```python
from build123d import *

# Parameters (mm, degrees)
SKETCH_1_W                = 54
SKETCH_1_H                = 220
EXTRUDE_1_DEPTH           = 30
SKETCH_2_W                = 42.2
SKETCH_2_H                = 48
CUT_EXTRUDE_1_DEPTH       = 25
SKETCH_3_W                = 42.2
SKETCH_3_H                = 46
CUT_EXTRUDE_2_DEPTH       = 25
CUT_EXTRUDE_3_DEPTH       = 6
CUT_EXTRUDE_13_DEPTH      = 6
SKETCH_18_W               = 32.2
SKETCH_18_H               = 32.2
CUT_EXTRUDE_9_DEPTH       = 6
SKETCH_9_R                = 15.6
SKETCH_9_R_2              = 1.6
CUT_EXTRUDE_4_DEPTH       = 25
SKETCH_16_W               = 42.7
SKETCH_16_H               = 42.7
CUT_EXTRUDE_7_DEPTH       = 2.5
SKETCH_13_R               = 20.35
SKETCH_13_R_2             = 2.1
CUT_EXTRUDE_6_DEPTH       = 28.5
EXTRUDE_3_DEPTH           = 30
SKETCH_17_R               = 1.5
CUT_EXTRUDE_8_DEPTH       = 8
SKETCH_21_R               = 3.5
CUT_EXTRUDE_11_DEPTH      = 1
CUT_EXTRUDE_11_DEPTH_BACK = 7.5
EXTRUDE_4_DEPTH           = 30
SKETCH_29_R               = 3
CUT_EXTRUDE_15_DEPTH      = 3
SKETCH_30_R               = 1.5
CUT_EXTRUDE_16_DEPTH      = 8


with BuildPart() as part:
    # 草图1 → 凸台-拉伸1 (new body)
    with BuildSketch(Plane.XY):
        Rectangle(SKETCH_1_W, SKETCH_1_H)
    extrude(amount=EXTRUDE_1_DEPTH)

    # 草图2 → 切除-拉伸1 (cut)
    with BuildSketch(Plane.XY.offset(30)):
        with Locations((0, 33)):
            Rectangle(SKETCH_2_W, SKETCH_2_H)
    extrude(amount=-CUT_EXTRUDE_1_DEPTH, mode=Mode.SUBTRACT)

    # 草图3 → 切除-拉伸2 (cut)
    with BuildSketch(Plane(origin=(0, 0, 30), x_dir=(-1, 0, 0), z_dir=(0, 0, -1))):
        with Locations((0, -33)):
            Rectangle(SKETCH_3_W, SKETCH_3_H)
    extrude(amount=CUT_EXTRUDE_2_DEPTH, mode=Mode.SUBTRACT)

    # 草图4 → 切除-拉伸3 (cut, through all)
    with BuildSketch(Plane.XY.offset(5)):
        with BuildLine():
            Line((11, 31), (11, 35))
            ThreePointArc((11, 35), (0, 46), (-11, 35))
            Line((-11, 35), (-11, 31))
            ThreePointArc((-11, 31), (0, 20), (11, 31))
        make_face()
        with BuildLine():
            Line((-14, 46.5), (-14, 50.5))
            ThreePointArc((-14, 50.5), (-15.5, 52), (-17, 50.5))
            Line((-17, 50.5), (-17, 46.5))
            ThreePointArc((-17, 46.5), (-15.5, 45), (-14, 46.5))
        make_face()
        with BuildLine():
            ThreePointArc((17, 50.5), (15.5, 52), (14, 50.5))
            Line((14, 50.5), (14, 46.5))
            ThreePointArc((14, 46.5), (15.5, 45), (17, 46.5))
            Line((17, 46.5), (17, 50.5))
        make_face()
        with BuildLine():
            Line((14, 19.5), (14, 15.5))
            ThreePointArc((14, 15.5), (15.5, 14), (17, 15.5))
            Line((17, 15.5), (17, 19.5))
            ThreePointArc((17, 19.5), (15.5, 21), (14, 19.5))
        make_face()
        with BuildLine():
            ThreePointArc((-17, 15.5), (-15.5, 14), (-14, 15.5))
            Line((-14, 15.5), (-14, 19.5))
            ThreePointArc((-14, 19.5), (-15.5, 21), (-17, 19.5))
            Line((-17, 19.5), (-17, 15.5))
        make_face()
    extrude(amount=-CUT_EXTRUDE_3_DEPTH, mode=Mode.SUBTRACT)

    # 草图26 → 切除-拉伸13 (cut, through all)
    with BuildSketch(Plane.XY.offset(5)):
        with BuildLine():
            Line((11, -31), (11, -35))
            ThreePointArc((11, -35), (0, -46), (-11, -35))
            Line((-11, -35), (-11, -31))
            ThreePointArc((-11, -31), (0, -20), (11, -31))
        make_face()
        with BuildLine():
            Line((-13.95, -15.5), (-13.95, -19.5))
            ThreePointArc((-13.95, -19.5), (-15.5, -21.05), (-17.05, -19.5))
            Line((-17.05, -19.5), (-17.05, -15.5))
            ThreePointArc((-17.05, -15.5), (-15.5, -13.95), (-13.95, -15.5))
        make_face()
        with BuildLine():
            Line((-13.95, -50.5), (-13.95, -46.5))
            ThreePointArc((-13.95, -46.5), (-15.5, -44.95), (-17.05, -46.5))
            Line((-17.05, -46.5), (-17.05, -50.5))
            ThreePointArc((-17.05, -50.5), (-15.5, -52.05), (-13.95, -50.5))
        make_face()
        with BuildLine():
            Line((13.95, -50.5), (13.95, -46.5))
            ThreePointArc((13.95, -46.5), (15.5, -44.95), (17.05, -46.5))
            Line((17.05, -46.5), (17.05, -50.5))
            ThreePointArc((17.05, -50.5), (15.5, -52.05), (13.95, -50.5))
        make_face()
        with BuildLine():
            Line((13.95, -15.5), (13.95, -19.5))
            ThreePointArc((13.95, -19.5), (15.5, -21.05), (17.05, -19.5))
            Line((17.05, -19.5), (17.05, -15.5))
            ThreePointArc((17.05, -15.5), (15.5, -13.95), (13.95, -15.5))
        make_face()
    extrude(amount=-CUT_EXTRUDE_13_DEPTH, mode=Mode.SUBTRACT)

    # 草图18 → 切除-拉伸9 (cut)
    with BuildSketch(Plane.XY):
        with Locations((0, -85)):
            Rectangle(SKETCH_18_W, SKETCH_18_H)
    extrude(amount=CUT_EXTRUDE_9_DEPTH, mode=Mode.SUBTRACT)

    # 草图9 → 切除-拉伸4 (cut, through all)
    with BuildSketch(Plane.XY.offset(6)):
        with Locations((0, -85)):
            Circle(SKETCH_9_R)
        with Locations((-13.258252147, -71.741747853)):
            Circle(SKETCH_9_R_2)
        with Locations((13.258252147, -71.741747853)):
            Circle(SKETCH_9_R_2)
        with Locations((13.258252147, -98.258252147)):
            Circle(SKETCH_9_R_2)
        with Locations((-13.258252147, -98.258252147)):
            Circle(SKETCH_9_R_2)
    extrude(amount=CUT_EXTRUDE_4_DEPTH, mode=Mode.SUBTRACT)

    # 草图16 → 切除-拉伸7 (cut)
    with BuildSketch(Plane.XY):
        with Locations((0, 85)):
            Rectangle(SKETCH_16_W, SKETCH_16_H)
    extrude(amount=CUT_EXTRUDE_7_DEPTH, mode=Mode.SUBTRACT)

    # 草图13 → 切除-拉伸6 (cut, through all)
    with BuildSketch(Plane(origin=(0, 0, 2.5), x_dir=(-1, 0, 0), z_dir=(0, 0, -1))):
        with Locations((0, 85)):
            Circle(SKETCH_13_R)
        with Locations((-17.67766953, 102.67766953)):
            Circle(SKETCH_13_R_2)
        with Locations((17.67766953, 102.67766953)):
            Circle(SKETCH_13_R_2)
        with Locations((17.67766953, 67.32233047)):
            Circle(SKETCH_13_R_2)
        with Locations((-17.67766953, 67.32233047)):
            Circle(SKETCH_13_R_2)
    extrude(amount=-CUT_EXTRUDE_6_DEPTH, mode=Mode.SUBTRACT)

    # 草图15 → 凸台-拉伸3 (add)
    with BuildSketch(Plane(origin=(0, 0, 0), x_dir=(-1, 0, 0), z_dir=(0, 0, -1))):
        with BuildLine():
            Line((-27, 110), (27, 110))
            ThreePointArc((27, 110), (0, 121.796738986), (-27, 110))
        make_face()
    extrude(amount=-EXTRUDE_3_DEPTH)

    # 草图17 → 切除-拉伸8 (cut)
    with BuildSketch(Plane(origin=(0, 0, 0), x_dir=(-1, 0, 0), z_dir=(0, 0, -1))):
        with Locations((-24, 100)):
            Circle(SKETCH_17_R)
        with Locations((24, 100)):
            Circle(SKETCH_17_R)
        with Locations((24, 66)):
            Circle(SKETCH_17_R)
        with Locations((-24, 66)):
            Circle(SKETCH_17_R)
    extrude(amount=-CUT_EXTRUDE_8_DEPTH, mode=Mode.SUBTRACT)

    # 草图21 → 切除-拉伸11 (cut, two sides)
    with BuildSketch(Plane.XY.offset(30)) as cut_extrude_11_sk:
        with Locations((-17.67766953, 102.67766953)):
            Circle(SKETCH_21_R)
        with Locations((17.67766953, 102.67766953)):
            Circle(SKETCH_21_R)
        with Locations((17.67766953, 67.32233047)):
            Circle(SKETCH_21_R)
        with Locations((-17.67766953, 67.32233047)):
            Circle(SKETCH_21_R)
    extrude(amount=CUT_EXTRUDE_11_DEPTH, mode=Mode.SUBTRACT)
    extrude(cut_extrude_11_sk.sketch, amount=-CUT_EXTRUDE_11_DEPTH_BACK, mode=Mode.SUBTRACT)

    # 草图28 → 凸台-拉伸4 (add)
    with BuildSketch(Plane.XY.offset(30)):
        with BuildLine():
            Line((-27, -110), (27, -110))
            ThreePointArc((27, -110), (0, -121.795200461), (-27, -110))
        make_face()
    extrude(amount=-EXTRUDE_4_DEPTH)

    # 草图29 → 切除-拉伸15 (cut)
    with BuildSketch(Plane.XY.offset(30)):
        with Locations((-13.258252147, -71.741747853)):
            Circle(SKETCH_29_R)
        with Locations((13.258252147, -71.741747853)):
            Circle(SKETCH_29_R)
        with Locations((13.258252147, -98.258252147)):
            Circle(SKETCH_29_R)
        with Locations((-13.258252147, -98.258252147)):
            Circle(SKETCH_29_R)
    extrude(amount=-CUT_EXTRUDE_15_DEPTH, mode=Mode.SUBTRACT)

    # 草图30 → 切除-拉伸16 (cut)
    with BuildSketch(Plane(origin=(0, 0, 0), x_dir=(-1, 0, 0), z_dir=(0, 0, -1))):
        with Locations((-24, -100)):
            Circle(SKETCH_30_R)
        with Locations((-24, -66)):
            Circle(SKETCH_30_R)
        with Locations((24, -66)):
            Circle(SKETCH_30_R)
        with Locations((24, -100)):
            Circle(SKETCH_30_R)
    extrude(amount=-CUT_EXTRUDE_16_DEPTH, mode=Mode.SUBTRACT)


solid = part.part
```
Part model, mm, in its own coordinate system. A direction names the side the tool comes from. Coordinates: 2 decimals unless noted, no trailing zeros. Loops run counter-clockwise (first coordinate to the right, second up) from the corner with the lowest first, then second, coordinate; pieces in that order, holes last. Notation, with made-up numbers: (-8.75, -14) - (39.25, -14) arc R7 ccw to (39.25, -3) - close; hole circle Ø5 at (78.25, 3.5). An arc over 180 degrees is marked (long way). Write item = value, one per line. Start each with the question number.
Item 1: Wall check: L1, parallel to X at y = -12, z = 24.25; L2, parallel to Y at x = 24, z = 2.5; L3, parallel to X at y = 100, z = 2.25. Give the ranges that are in metal, low to high. Write a range as from..to.
Item 2: Flat gauge pins, fed straight in: pin 1 Ø8 at (x, y) = (13.26, -98.26) entering from -Z; pin 2 Ø0.9 at (x, y) = (-23.5, 66.5) entering from -Z; pin 3 Ø2 at (x, z) = (20, 4) entering from -Y; pin 4 Ø2 at (x, z) = (-9, 19) entering from -Y. Where does each tip first touch, or does it go through?
Item 3: Cut at A-A, the plane y = 76. Give the cut face in (x, z).
Item 4: 3-axis set-ups, long thin cutter, end or side, ignore diameter. For faces 1 (the cylindrical face through (11.05, -69.71, 28.52)), 2 (the flat face through (0, 2, 30)), 3 (the flat face through (-17, 18, 3)), 4 (the flat face through (-8, 66, 2.5)): which of +Z, -Z, +X, -X, +Y, -Y reach the whole face in a straight line?
Item 5: Cut at C-C, the plane y = -25. Give the cut face in (x, z), and give its area (3 significant figures).
Item 6: Cut at B-B, the plane x = 2. State how many separate pieces and enclosed holes the cut face has, and give its area (3 significant figures).
Item 7: Mould opens along X. For faces 5 (the cylindrical face through (0.424, -121.793, 15.21)), 6 (the flat face through (0, 2, 0)), 7 (the cylindrical face through (-15.469, -69.714, 28.521)) say: released by +X, released by -X, zero draft, split by the parting line, or undercut.
The answers:
q1.L1 = -27..-21.1, 21.1..27
q1.L2 = -112.89..-101.5, -98.5..-67.5, -64.5..64.5, 67.5..98.5, 101.5..112.89
q1.L3 = -27..-25.5, -22.5..-21.35, 21.35..22.5, 25.5..27
q2.pin_1 = 0
q2.pin_2 = 8
q2.pin_3 = -116.51
q2.pin_4 = -120.92
q3.outline = (-27, 0) - (-21.35, 0) - (-21.35, 2.5) - (-18.25, 2.5) - (-18.25, 30) - (-27, 30) - close; (18.25, 2.5) - (21.35, 2.5) - (21.35, 0) - (27, 0) - (27, 30) - (18.25, 30) - close
q4.face_1 = +Z
q4.face_2 = +Z, +X, -X, +Y, -Y
q4.face_3 = +Z, -Z
q4.face_4 = -Z
q5.outline = (-27, 0) - (-9.22, 0) - (-9.22, 5) - (-21.1, 5) - (-21.1, 30) - (-27, 30) - close; (9.22, 0) - (27, 0) - (27, 30) - (21.1, 30) - (21.1, 5) - (9.22, 5) - close
q5.area = 473 mm2
q6.separate_pieces = 5
q6.enclosed_holes = 0
q6.area = 2,540 mm2
q7.face_5 = split by the parting line
q7.face_6 = zero draft
q7.face_7 = undercut
